For this review, take the finished solid that the model builds, in its own axes (mm). A direction names the side the tool comes from. Give positions to 0.01 mm unless a question says otherwise; leave off trailing zeros. Order: outer loops, then holes, each group sorted by start corner. A loop starts at its lowest first (then second) coordinate and runs counter-clockwise, first axis right, second up.
from build123d import *

# Parameters (mm, degrees)
SCHIZZO1_W                = 135
SCHIZZO1_H                = 135
SCHIZZO1_R                = 5.5
ESTRUSIONE1_DEPTH         = 16
SCHIZZO2_W                = 62
SCHIZZO2_H                = 62
ESTRUSIONE_SOTTILE1_DEPTH = 205
SCHIZZO3_W                = 321.5
SCHIZZO3_H                = 110
ESTRUSIONE2_DEPTH         = 30
SCHIZZO4_R                = 40
ESTRUSIONE3_DEPTH         = 270
SCHIZZO6_R                = 32
ESTRUSIONE4_DEPTH         = 642.456935421
SCHIZZO7_R                = 35
ESTRUSIONE5_DEPTH         = 28
ESTRUSIONE6_START         = -28
SCHIZZO8_R                = 35
ESTRUSIONE6_DEPTH         = 28
SCHIZZO9_W                = 80
SCHIZZO9_H                = 16
ESTRUSIONE7_DEPTH         = 85
SCHIZZO10_R               = 16
ESTRUSIONE8_DEPTH         = 40
SCHIZZO11_R               = 17.5
ESTRUSIONE9_DEPTH         = 40
SMUSSO1_SIZE              = 15
SCHIZZO12_R               = 37
ESTRUSIONE10_DEPTH        = 8
ESTRUSIONE11_START        = -8
SCHIZZO13_R               = 37
ESTRUSIONE11_DEPTH        = 8
M16_TAPPED_HOLE1_D        = 14
M16_TAPPED_HOLE1_DEPTH    = 42
M16_TAPPED_HOLE1_TIP      = 4.206024333


with BuildPart() as part:
    # Schizzo1 → Estrusione1 (new body)
    with BuildSketch(Plane(origin=(0, 0, 0), x_dir=(1, 0, 0), z_dir=(0, 1, 0))):
        with Locations((67.5, 67.5)):
            Rectangle(SCHIZZO1_W, SCHIZZO1_H)
        with Locations(Location((22.5, 112.5, 0), (0, 0, 270))):
            Circle(SCHIZZO1_R, mode=Mode.SUBTRACT)
        with Locations(Location((112.5, 112.5, 0), (0, 0, 90))):
            Circle(SCHIZZO1_R, mode=Mode.SUBTRACT)
        with Locations(Location((112.5, 22.5, 0), (0, 0, 270))):
            Circle(SCHIZZO1_R, mode=Mode.SUBTRACT)
        with Locations(Location((22.5, 22.5, 0), (0, 0, 90))):
            Circle(SCHIZZO1_R, mode=Mode.SUBTRACT)
    extrude(amount=ESTRUSIONE1_DEPTH)

    # Schizzo2 → Estrusione-Sottile1 (add)
    with BuildSketch(Plane.XZ):
        with BuildLine():
            Line((32.5, -99.5), (32.5, -35.5))
            ThreePointArc((32.5, -35.5), (33.378679656, -33.378679656), (35.5, -32.5))
            Line((35.5, -32.5), (99.5, -32.5))
            ThreePointArc((99.5, -32.5), (101.621320344, -33.378679656), (102.5, -35.5))
            Line((102.5, -35.5), (102.5, -99.5))
            ThreePointArc((102.5, -99.5), (101.621320344, -101.621320344), (99.5, -102.5))
            Line((99.5, -102.5), (35.5, -102.5))
            ThreePointArc((35.5, -102.5), (33.378679656, -101.621320344), (32.5, -99.5))
        make_face()
        with Locations((67.5, -67.5)):
            Rectangle(SCHIZZO2_W, SCHIZZO2_H, mode=Mode.SUBTRACT)
    extrude(amount=ESTRUSIONE_SOTTILE1_DEPTH)

    # Schizzo3 → Estrusione2 (add)
    with BuildSketch(Plane.XZ.offset(205)):
        with Locations((188.25, -67.5)):
            Rectangle(SCHIZZO3_W, SCHIZZO3_H)
    extrude(amount=ESTRUSIONE2_DEPTH)

    # Schizzo4 → Estrusione3 (add)
    with BuildSketch(Plane.XZ.offset(235)):
        with Locations(Location((304, -67.5, 0), (0, 0, 270))):
            Circle(SCHIZZO4_R)
    extrude(amount=ESTRUSIONE3_DEPTH)

    # Schizzo6 → Estrusione4 (cut, through all)
    with BuildSketch(Plane.XZ.offset(505)):
        with Locations(Location((304, -67.5, 0), (0, 0, 270))):
            Circle(SCHIZZO6_R)
    extrude(amount=-ESTRUSIONE4_DEPTH, mode=Mode.SUBTRACT)

    # Schizzo7 → Estrusione5 (cut)
    with BuildSketch(Plane.XZ.offset(505)):
        with Locations(Location((304, -67.5, 0), (0, 0, 270))):
            Circle(SCHIZZO7_R)
    extrude(amount=-ESTRUSIONE5_DEPTH, mode=Mode.SUBTRACT)

    # Schizzo8 → Estrusione6 (cut)
    with BuildSketch(Plane(origin=(0, -205, 0), x_dir=(1, 0, 0), z_dir=(0, 1, 0)).offset(ESTRUSIONE6_START)):
        with Locations(Location((304, 67.5, 0), (0, 0, 90))):
            Circle(SCHIZZO8_R)
    extrude(amount=ESTRUSIONE6_DEPTH, mode=Mode.SUBTRACT)

    # Schizzo9 → Estrusione7 (add)
    with BuildSketch(Plane.XZ.offset(235)):
        with Locations((67.5, -114.5)):
            Rectangle(SCHIZZO9_W, SCHIZZO9_H)
        with Locations((67.5, -20.5)):
            Rectangle(SCHIZZO9_W, SCHIZZO9_H)
    extrude(amount=ESTRUSIONE7_DEPTH)

    # Schizzo10 → Estrusione8 (cut)
    with BuildSketch(Plane.XY.offset(-12.5)):
        with Locations((67.5, -290)):
            Circle(SCHIZZO10_R)
    extrude(amount=-ESTRUSIONE8_DEPTH, mode=Mode.SUBTRACT)

    # Schizzo11 → Estrusione9 (cut)
    with BuildSketch(Plane(origin=(0, 0, -122.5), x_dir=(-1, 0, 0), z_dir=(0, 0, -1))):
        with Locations((-67.5, -290)):
            Circle(SCHIZZO11_R)
    extrude(amount=-ESTRUSIONE9_DEPTH, mode=Mode.SUBTRACT)

    # Smusso1
    smusso1_edges = [part.edges().sort_by_distance(p)[0] for p in [
        (27.5, -320, -20.5),
        (107.5, -320, -20.5),
        (107.5, -320, -114.5),
        (27.5, -320, -114.5),
        (349, -220, -122.5),
        (349, -220, -12.5),
    ]]
    chamfer(smusso1_edges, length=SMUSSO1_SIZE)

    # Schizzo12 → Estrusione10 (cut)
    with BuildSketch(Plane.XZ.offset(505)):
        with Locations(Location((304, -67.5, 0), (0, 0, 270))):
            Circle(SCHIZZO12_R)
    extrude(amount=-ESTRUSIONE10_DEPTH, mode=Mode.SUBTRACT)

    # Schizzo13 → Estrusione11 (cut)
    with BuildSketch(Plane(origin=(0, -205, 0), x_dir=(1, 0, 0), z_dir=(0, 1, 0)).offset(ESTRUSIONE11_START)):
        with Locations(Location((304, 67.5, 0), (0, 0, 90))):
            Circle(SCHIZZO13_R)
    extrude(amount=ESTRUSIONE11_DEPTH, mode=Mode.SUBTRACT)

    # M16 Tapped Hole1
    with Locations(Plane(origin=(0, 16, 0), x_dir=(-1, 0, 0), z_dir=(0, 1, 0))):
        with Locations((-67.5, -123), (-12, -67.5), (-67.5, -12), (-123, -67.5)):
            Hole(M16_TAPPED_HOLE1_D / 2, depth=M16_TAPPED_HOLE1_DEPTH)
            with Locations((0, 0, -(M16_TAPPED_HOLE1_DEPTH + M16_TAPPED_HOLE1_TIP / 2))):  # 118° drill point
                Cone(0, M16_TAPPED_HOLE1_D / 2, M16_TAPPED_HOLE1_TIP, mode=Mode.SUBTRACT)


solid = part.part
1) Draft analysis for pull direction X (two halves, no side actions). For faces 1 (the face through (0, 8, -67)), 2 (the face through (349, -220, -68)), 3 (the face through (11.09, 7.89, -60.56)), state which applies: +X half, -X half, draft (parallel to the pull), parting line (faces both ways), or undercut.
Answer sheet:
face 1: -X half
face 2: +X half
face 3: undercut
2) To check wall thickness, follow line 1 (Z direction, x = 94, y = -182.5); line 2 (Y direction, x = 124.5, z = -77.5); line 3 (X direction, y = 10, z = -112.5). State the ranges of each line that lie inside material, in increasing order.
Answer sheet:
line 1: z = -102.5 to -98.5, -36.5 to -32.5
line 2: y = -235 to -205, 0 to 16
line 3: x = 0 to 17, 28 to 107, 118 to 135
3) We need section D-D on x = 201.5. Give the boundary of the cut face in (y, z), then the cut area to 3 significant figures.
Answer sheet:
outline: (-235, -122.5) - (-205, -122.5) - (-205, -12.5) - (-235, -12.5) - close
area: 3,300 mm2
4) We need section B-B on y = -158. Give the boundary of the cut face in (x, z).
Answer sheet:
outline: (32.5, -99.5) arc R3 ccw to (35.5, -102.5) - (99.5, -102.5) arc R3 ccw to (102.5, -99.5) - (102.5, -35.5) arc R3 ccw to (99.5, -32.5) - (35.5, -32.5) arc R3 ccw to (32.5, -35.5) - close; hole (36.5, -98.5) - (98.5, -98.5) - (98.5, -36.5) - (36.5, -36.5) - close
5) Tool access review of faces 4 (the face through (67, 0, -113)), 5 (the face through (27.5, -232, -68)), 6 (the face through (117.953, 7.888, -23.216)), 7 (the face through (145, -223, -12.5)): name each direction out of +Z, -Z, +X, -X, +Y, -Y from which nothing blocks a thin tool from reaching the whole face with its end or side.
Answer sheet:
face 4: none
face 5: +Z, -Z, -X, -Y
face 6: +Y
face 7: +Z, +X, -X, -Y
6) Clearance check with flat-ended pins moving along their axes: pin 1 (2 mm diameter, centred on y = -244.5, z = -66.5, fed in from -X); pin 2 (5 mm diameter, centred on x = 259.5, z = -43.5, fed in from +Y); pin 3 (8 mm diameter, centred on y = -164, z = -52, fed in from -X). State where each tip first meets the part, or that it passes through.
Answer sheet:
pin 1: stops at x = 264
pin 2: stops at y = -205
pin 3: stops at x = 32.5
7) We need section A-A on x = 304. Give the boundary of the cut face in (y, z).
Answer sheet:
outline: (-505, -107.5) - (-235, -107.5) - (-235, -122.5) - (-205, -122.5) - (-205, -104.5) - (-213, -104.5) - (-213, -102.5) - (-233, -102.5) - (-233, -99.5) - (-477, -99.5) - (-477, -102.5) - (-497, -102.5) - (-497, -104.5) - (-505, -104.5) - close; (-505, -30.5) - (-497, -30.5) - (-497, -32.5) - (-477, -32.5) - (-477, -35.5) - (-233, -35.5) - (-233, -32.5) - (-213, -32.5) - (-213, -30.5) - (-205, -30.5) - (-205, -12.5) - (-235, -12.5) - (-235, -27.5) - (-505, -27.5) - close
8) We need section C-C on z = -67.5. Count the separate pieces of the cut face and the enclosed holes in it, then the cut area to 3 significant figures.
Answer sheet:
separate pieces: 4
enclosed holes: 1
area: 15,000 mm2
